The model under review builds one solid part; all positions refer to its coordinate system, in mm. A direction names the side the tool comes from. Round coordinates to 2 decimals unless told otherwise and drop trailing zeros. Loops run counter-clockwise (first coordinate to the right, second up) from the corner with the lowest first, then second, coordinate; pieces in that order, holes last. Notation, with made-up numbers: (40.5, -33.5) - (53.5, -33.5) arc R19 cw to (53.5, -18.5) - close; hole circle Ø6 at (42, -25). An arc over 180 degrees is marked (long way). Answer as CSV lines item,"result".
Solid Edge part; units mm, degrees
sketch "Sketch1" plane through (0, 0, 0) normal (0, -1, 0) x (1, 0, 0)
  line L0 (0, 40) -> (0, -40)
  arc A0 (0, 40) -> (0, -40) centre (0, 0) cw
revolve "RevolvedProtrusion1" add sketch "Sketch1" angle 360 about axis through (0, 0, 45) along (0, 0, -1)
sketch "Sketch2" plane through (0, 0, 0) normal (0, 0, 1) x (1, 0, 0)
  circle A0 centre (0, 0) radius 5.09
extrude "Protrusion1" add sketch "Sketch2" against normal blind 55
sketch "Sketch3" plane through (0, 0, -55) normal (0, 0, -1) x (1, 0, 0)
  line L0 (-24, 0) -> (-12, -20.7846)
  line L1 (-12, -20.7846) -> (12, -20.7846)
  line L2 (12, -20.7846) -> (24, 0)
  line L3 (24, 0) -> (12, 20.7846)
  line L4 (12, 20.7846) -> (-12, 20.7846)
  line L5 (-12, 20.7846) -> (-24, 0)
extrude "ExtrudedProtrusion_3" add sketch "Sketch3" along normal blind 4
shell "Thinwall_1" thickness 0 removed faces 1 at (16.48, 0.4157, -59) outside thickness 1
1. Wall thickness on probe 1 along Y at (x, z) = (0, -44); probe 2 along Z at (x, y) = (-6, 14); probe 3 along Z at (x, y) = (-12.5, -17): over which ranges is each line inside the solid? List them lowest first.
Numbers:
probe 1,"y = -6.09 to -5.09, 5.09 to 6.09"
probe 2,"z = -55 to -54, -38.07 to -36.99, 36.99 to 38.07"
probe 3,"z = -55 to -54, -35.15 to -33.98, 33.98 to 35.15"
2. Clearance check with flat-ended pins moving along their axes: pin 1 (3 mm diameter, centred on x = -14.5, y = -28, fed in from -Z); pin 2 (21 mm diameter, centred on x = 3, y = 1, fed in from -Z); pin 3 (2 mm diameter, centred on x = 6, z = -57.5, fed in from +Y). State where each tip first meets the part, or that it passes through.
Numbers:
pin 1,"stops at z = -27.91"
pin 2,"stops at z = -55"
pin 3,"stops at y = 21.78"
3. Take a section at A-A (x = -14). State the section outline as (y, z) points, plus the area to 3 significant figures.
Numbers:
outline,"circle Ø77.07 at (0, 0); (-19.32, -59) - (-17.32, -59) - (-17.32, -55) - (17.32, -55) - (17.32, -59) - (19.32, -59) - (19.32, -54) - (-19.32, -54) - close; hole circle Ø74.94 at (0, 0)"
area,"309 mm²"
4. Take a section at D-D (y = 31.5). State the section outline as (x, z) points, plus the area to 3 significant figures.
Numbers:
outline,"circle Ø52.49 at (0, 0); hole circle Ø49.31 at (0, 0)"
area,"254 mm²"
5. Draft analysis for pull direction Y (two halves, no side actions). For faces 5 (the face through (-17.916, -10.538, -56.972)), 6 (the face through (-19, 10, -59)), 7 (the face through (18.954, -10.74, -56.465)), 8 (the face through (0, 20.785, -57)), state which applies: +Y half, -Y half, draft (parallel to the pull), parting line (faces both ways), or undercut.
Numbers:
face 5,"undercut"
face 6,"draft"
face 7,"-Y half"
face 8,"undercut"
6. Tool access review of faces 1 (the face through (-18.954, 10.74, -56.465)), 2 (the face through (0, 21.785, -56)), 3 (the face through (18.08, -10.25, -56.97)), 4 (the face through (18.78, 11.04, -56.46)): name each direction out of +Z, -Z, +X, -X, +Y, -Y from which nothing blocks a thin tool from reaching the whole face with its end or side.
Numbers:
face 1,"-Z, -X, +Y"
face 2,"-Z, +X, -X, +Y"
face 3,"-Z"
face 4,"-Z, +X, +Y"
7. Take a section at C-C (z = -28.5). State the section outline as (x, y) points.
Numbers:
outline,"circle Ø58.95 at (0, 0); hole circle Ø56.13 at (0, 0)"
8. Take a section at B-B (x = 0). State the section outline as (y, z) points, plus the area to 3 significant figures.
Numbers:
outline,"(-21.78, -59) - (-20.78, -59) - (-20.78, -55) - (-5.09, -55) - (-5.09, -39.67) arc R40 cw (long way) to (5.09, -39.67) - (5.09, -55) - (20.78, -55) - (20.78, -59) - (21.78, -59) - (21.78, -54) - (6.09, -54) - (6.09, -40.55) arc R41 ccw (long way) to (-6.09, -40.55) - (-6.09, -54) - (-21.78, -54) - close"
area,"312 mm²"
